Design review of the part built by this model. Coordinates are the model's own, in mm. A direction names the side the tool comes from. Give positions to 0.01 mm unless a question says otherwise; leave off trailing zeros. Write each loop counter-clockwise with the first axis right and the second up, starting at its lowest first coordinate (ties: lowest second). Pieces come first, ordered by that corner, then holes. Notation, with made-up numbers: M 76.25,74.25 L 109.25,74.25 A33 cw 109.25,113.25 Z; hole C 16,-30.5 d11. An arc over 180 degrees is marked long. Answer in a Markdown table with one row per item.
Solid Edge part; units mm, degrees
sketch "Sketch1" plane through (0, 0, 0) normal (0, -1, 0) x (1, 0, 0)
  line L0 (0, -20) -> (4, -20)
  line L1 (4, -20) -> (4, -1.237)
  line L2 (4, -1.237) -> (3.594, -0.425)
  line L3 (3.594, -0.425) -> (3.594, 0)
  line L4 (3.594, 0) -> (7.5056, 0)
  line L5 (7.5056, 0) -> (7.5056, 5.3)
  line L6 (7.5056, 5.3) -> (0, 5.3)
  dimension "D1" = 3.594
  dimension "D2" = 4
  dimension "D3" = 7.5056
revolve "RevolvedProtrusion1" add sketch "Sketch1" angle 360 about axis through (0, 0, 6.4) along (0, 0, -1)
sketch "Sketch2" plane through (0, 0, 0) normal (0, 0, 1) x (1, 0, 0)
  line L0 (7.5056, 0) -> (3.7528, 6.5)
  arc A0 (3.7528, 6.5) -> (7.5056, 0) centre (0, 0) cw
extrude "ExtrudedCutout_1" cut sketch "Sketch2" along normal blind 5.3
pattern_circular "Pattern1" count 6 over 360 about axis through (0, 0, 5.3) along (0, 0, 1) of "ExtrudedCutout_1"
sketch "Sketch3" plane through (0, 0, 0) normal (0, -1, 0) x (1, 0, 0)
  line L0 (5.815, 0) -> (5.815, 0.6)
  line L1 (5.815, 0.6) -> (7.5056, 0.6)
  line L2 (7.5056, 0.6) -> (7.5056, 0)
  line L3 (7.5056, 0) -> (5.815, 0)
  line L4 (6.4875, 5.3) -> (7.5056, 5.3)
  line L5 (7.5056, 5.3) -> (7.5056, 4.7122)
  line L6 (7.5056, 4.7122) -> (6.4875, 5.3)
  dimension "D1" = 6.4875
  dimension "D2" = 7.5056
revolve "RevolvedCutout_1" cut sketch "Sketch3" angle 360 about axis through (0, 0, 6.4) along (0, 0, -1)
cosmetic_thread "Thread_1" thread depth 18.763
chamfer "Chamfer_1" distance 0.767 angle 45 1 edges at (-4, 0, -20) measured on face at (2.7467, 2.5867, -20)
fillet "Round_1" radius 0.4 1 edges at (-3.594, 0, 0)
fillet "Round_2" radius 0.15 1 edges at (-5.815, 0, 0)
fillet "Round_3" radius 0.4475 1 edges at (-5.815, 0, 0.6)
properties material "Steel"
1) Insertion check: P1, Ø5, axis at y = 2.5, z = -15.5, coming from the +X side; P2, Ø8, axis at x = 5, z = -4.5, coming from the -Y side; P3, Ø1, axis at x = 2, z = -13.5, coming from the +Y side. Each pin has a flat end and moves straight along its axis. Give the tip position at first contact, or say it passes through.
Geometry says:
| item | result |
|---|---|
| P1 | x = 4 |
| P2 | y = -3.87 |
| P3 | y = 3.71 |
2) To check wall thickness, follow probe 1 along Y at (x, z) = (0.25, -11.5); probe 2 along Z at (x, y) = (2.5, -5); probe 3 along X at (y, z) = (0, -1.5). State the ranges of each line that lie inside material, in increasing order. Write a range as [from, to].
Geometry says:
| item | result |
|---|---|
| probe 1 | [-3.99, 3.99] |
| probe 2 | [0, 5.3] |
| probe 3 | [-4, 4] |
3) Add section B-B (z = -3). Write out the cut boundary in (x, y), and give its area (3 significant figures).
Geometry says:
| item | result |
|---|---|
| outline | C 0,0 d8 |
| area | 50.3 mm^2 |
4) For faces 1 (the face through (0, 0, -20)), 2 (the face through (-0.867, -3.905, -10.109)), list the 3-axis set-ups (+Z, -Z, +X, -X, +Y, -Y) from which the entire face can be reached by the end or side of a thin tool; tool diameter is ignored.
Geometry says:
| item | result |
|---|---|
| face 1 | -Z, +X, -X, +Y, -Y |
| face 2 | -Z |
